```python
from build123d import *

# Parameters (mm, degrees)
SKETCH1_W           = 40
SKETCH1_H           = 19.5
BOSS_EXTRUDE1_DEPTH = 23.625
SKETCH2_R           = 6.1
CUT_EXTRUDE1_DEPTH  = 36.25
CUT_EXTRUDE2_REACH  = 49.46
SKETCH3_R           = 5
SKETCH5_R           = 3
CUT_EXTRUDE3_DEPTH  = 18
CUT_EXTRUDE4_REACH  = 50.003
SKETCH6_R           = 1.25
SKETCH7_R           = 1.25
CUT_EXTRUDE5_DEPTH  = 6.75
FILLET1_R           = 2
FILLET2_DEPTH       = 23.625


with BuildPart() as part:
    # Sketch1 → Boss-Extrude1 (new body)
    with BuildSketch(Plane(origin=(0, 0, 0), x_dir=(1, 0, 0), z_dir=(0, 1, 0))):
        with Locations((20, 9.75)):
            Rectangle(SKETCH1_W, SKETCH1_H)
    extrude(amount=BOSS_EXTRUDE1_DEPTH)

    # Sketch2 → Cut-Extrude1 (cut)
    with BuildSketch(Plane(origin=(40, 0, 0), x_dir=(0, 0, -1), z_dir=(1, 0, 0))):
        with Locations((9.75, 9.3125)):
            Circle(SKETCH2_R)
    extrude(amount=-CUT_EXTRUDE1_DEPTH, mode=Mode.SUBTRACT)

    # Sketch3 → Cut-Extrude2 (cut, up to next)
    with BuildSketch(Plane(origin=(3.75, 0, 0), x_dir=(0, 0, -1), z_dir=(1, 0, 0)), mode=Mode.PRIVATE) as cut_extrude2_sk1:
        with Locations((9.75, 9.3125)):
            Circle(SKETCH3_R)
    cut_extrude2_tool1 = extrude(cut_extrude2_sk1.sketch, amount=-CUT_EXTRUDE2_REACH, mode=Mode.PRIVATE) & part.part
    add(cut_extrude2_tool1.solids().sort_by_distance((3.75, 9.3125, -9.75))[0], mode=Mode.SUBTRACT)

    # Sketch5 → Cut-Extrude3 (cut)
    with BuildSketch(Plane.XZ):
        with Locations(Location((34.25, -9.75, 0), (0, 0, 270))):
            Circle(SKETCH5_R)
        with Locations(Location((10.5, -9.75, 0), (0, 0, 270))):
            Circle(SKETCH5_R)
    extrude(amount=-CUT_EXTRUDE3_DEPTH, mode=Mode.SUBTRACT)

    # Sketch6 → Cut-Extrude4 (cut, up to next)
    with BuildSketch(Plane.XZ.offset(-18), mode=Mode.PRIVATE) as cut_extrude4_sk1:
        with Locations(Location((10.5, -9.75, 0), (0, 0, 270))):
            Circle(SKETCH6_R)
    cut_extrude4_tool1 = extrude(cut_extrude4_sk1.sketch, amount=-CUT_EXTRUDE4_REACH, mode=Mode.PRIVATE) & part.part
    # Sketch6 → Cut-Extrude4 (cut, up to next)
    with BuildSketch(Plane.XZ.offset(-18), mode=Mode.PRIVATE) as cut_extrude4_sk2:
        with Locations(Location((34.25, -9.75, 0), (0, 0, 270))):
            Circle(SKETCH6_R)
    cut_extrude4_tool2 = extrude(cut_extrude4_sk2.sketch, amount=-CUT_EXTRUDE4_REACH, mode=Mode.PRIVATE) & part.part
    add(cut_extrude4_tool1.solids().sort_by_distance((10.5, 18, -9.75))[0], mode=Mode.SUBTRACT)
    add(cut_extrude4_tool2.solids().sort_by_distance((34.25, 18, -9.75))[0], mode=Mode.SUBTRACT)

    # Sketch7 → Cut-Extrude5 (cut)
    with BuildSketch(Plane.XZ):
        with Locations(Location((20, -3, 0), (0, 0, 270))):
            Circle(SKETCH7_R)
        with Locations(Location((20, -16.5, 0), (0, 0, 270))):
            Circle(SKETCH7_R)
    extrude(amount=-CUT_EXTRUDE5_DEPTH, mode=Mode.SUBTRACT)

    # Fillet1
    fillet1_edges = [part.edges().sort_by_distance(p)[0] for p in [
        (40, 9.3125, -3.65),
    ]]
    fillet(fillet1_edges, radius=FILLET1_R)

    # Fillet2: read off the stored shape, not the designer's step
    # Fillet2 outline → Fillet2 (cut)
    with BuildSketch(Plane(origin=(0, 0, 0), x_dir=(1, 0, 0), z_dir=(0, 1, 0))):
        with BuildLine():
            Line((0, 19.5), (0, 9.75))
            ThreePointArc((0, 9.75), (2.855708883, 16.644291117), (9.75, 19.5))
            Line((9.75, 19.5), (0, 19.5))
        make_face()
        with BuildLine():
            ThreePointArc((9.75, 0), (2.855708883, 2.855708883), (0, 9.75))
            Line((0, 9.75), (0, 0))
            Line((0, 0), (9.75, 0))
        make_face()
    extrude(amount=FILLET2_DEPTH, mode=Mode.SUBTRACT)


solid = part.part
```
CAD build for the part. Positions are in the model's coordinates, mm. A direction names the side the tool comes from. Give positions to 0.01 mm unless a question says otherwise; leave off trailing zeros. Loops run counter-clockwise (first coordinate to the right, second up) from the corner with the lowest first, then second, coordinate; pieces in that order, holes last. Notation, with made-up numbers: (-32, 17.5) -> (-1, 17.5) arc R20 ccw to (-1, 30.5) -> close; hole circle Ø3 at (46.25, -30). An arc over 180 degrees is marked (long way). Use a Markdown table: item, result.
1. Flat gauge pins, fed straight in: pin 1 (5.5 mm diameter, centred on x = 34.25, z = -9.75, fed in from -Y); pin 2 (10 mm diameter, centred on x = 34, y = 2.5, fed in from +Z); pin 3 (0.7 mm diameter, centred on x = 19.5, z = -2.5, fed in from -Y); pin 4 (10 mm diameter, centred on y = 7.5, z = -10, fed in from +X). Where does each tip first touch, or does it go through?
Check result:
| item | result |
|---|---|
| pin 1 | stops at y = 18 |
| pin 2 | stops at z = 0 |
| pin 3 | stops at y = 6.75 |
| pin 4 | stops at x = 39.54 |
2. Slice it at D-D (z = -8). Give the number of separate pieces and of enclosed holes in the cut face, plus the area to 3 significant figures.
Check result:
| item | result |
|---|---|
| separate pieces | 4 |
| enclosed holes | 0 |
| area | 421 mm^2 |
3. Slice it at A-A (y = 19). List the corners of the cut face in (x, z).
Check result:
| item | result |
|---|---|
| outline | (9.75, -19.5) -> (40, -19.5) -> (40, 0) -> (9.75, 0) arc R9.75 ccw to start; hole circle Ø2.5 at (10.5, -9.75); hole circle Ø2.5 at (34.25, -9.75) |
4. Wall check: L1, parallel to X at y = 20.85, z = -9.75; L2, parallel to Y at x = 3, z = -10 (3 decimals); L3, parallel to Z at x = 10.5, y = 2.65. Give the ranges that are in metal, low to high. Write a range as [from, to].
Check result:
| item | result |
|---|---|
| L1 | x = [0, 9.25], [11.75, 33], [35.5, 40] |
| L2 | y = [0, 4.319], [14.306, 23.625] |
| L3 | z = [-19.5, -12.75], [-6.75, 0] |
5. Which spindle directions (+Z, -Z, +X, -X, +Y, -Y) get a long thin tool onto all of the face, cutting with end or side? Do faces 1 (the flat face through (3.75, 12, -5)), 2 (the flat face through (25, 12, -19.5)), 3 (the flat face through (33, 18, -10.4)). Say none if no direction does.
Check result:
| item | result |
|---|---|
| face 1 | +X |
| face 2 | -Z, +X, -X, +Y, -Y |
| face 3 | -Y |
6. Mould opens along X. For faces 4 (the flat face through (40, 17, -5)), 5 (the flat face through (20, 23.625, -10)), 6 (the flat face through (9, 18, -10)) say: pulls with the +X half, pulls with the -X half, needs draft (parallel to the pull), parting line crosses it, or undercut.
Check result:
| item | result |
|---|---|
| face 4 | pulls with the +X half |
| face 5 | needs draft |
| face 6 | undercut |
